```python
from build123d import *

# Parameters (mm, degrees)
SKETCH1_W                = 222.53
SKETCH1_H                = 140
TOP_PLATE_DEPTH          = 6
CORNER_FILLET_R          = 5
M3_CLEARANCE_HOLE1_D     = 3.4
M3_CLEARANCE_HOLE1_DEPTH = 4.228536948
M3_CLEARANCE_HOLE1_TIP   = 1.021463052
SKETCH4_R                = 16.25
SKETCH4_R_2              = 13.25
PRIMARY_BUTTONS_DEPTH    = 10
EXTRA_BUTTONS_REACH      = 8
SKETCH8_W                = 207.53
SKETCH8_H                = 125
HOLLOW_OUT_DEPTH         = 3.3
FILLET1_R                = 10
FILLET2_R                = 5
SKETCH15_W               = 64
SKETCH15_H               = 16
CUT_EXTRUDE4_DEPTH       = 4.4
LIGHT_GUIDE_CUTOUT_DEPTH = 10
CHAMFER1_SIZE            = 1
TOP_CHAMFER_SIZE         = 1.5
NUT_START                = -1.2
NUT_CUTOUT_DEPTH         = 2


with BuildPart() as part:
    # Sketch1 → Top Plate (new body)
    with BuildSketch(Plane(origin=(0, 0, 0), x_dir=(1, 0, 0), z_dir=(0, 1, 0))):
        with Locations((111.265, 70)):
            Rectangle(SKETCH1_W, SKETCH1_H)
    extrude(amount=TOP_PLATE_DEPTH)

    # Corner Fillet
    corner_fillet_edges = [part.edges().sort_by_distance(p)[0] for p in [
        (0, 3, -140),
        (222.53, 3, -140),
        (222.53, 3, 0),
        (0, 3, 0),
    ]]
    fillet(corner_fillet_edges, radius=CORNER_FILLET_R)

    # M3 Clearance Hole1
    with Locations(Plane(origin=(217.03, 0, -5.5), x_dir=(0, 0, -1), z_dir=(0, -1, 0))):
        with Locations((0, 0), (129, 0), (129, -211.53), (0, -211.53)):
            Hole(M3_CLEARANCE_HOLE1_D / 2, depth=M3_CLEARANCE_HOLE1_DEPTH)
            with Locations((0, 0, -(M3_CLEARANCE_HOLE1_DEPTH + M3_CLEARANCE_HOLE1_TIP / 2))):  # 118° drill point
                Cone(0, M3_CLEARANCE_HOLE1_D / 2, M3_CLEARANCE_HOLE1_TIP, mode=Mode.SUBTRACT)

    # Sketch4 → Primary Buttons (cut)
    with BuildSketch(Plane(origin=(0, 6, 0), x_dir=(-1, 0, 0), z_dir=(0, -1, 0))):
        with BuildLine():
            ThreePointArc((-48.971318984, 103.179989332), (-49.620754304, 103.829424652), (-50.539194542, 103.829424652))
            Line((-50.539194542, 103.829424652), (-67.030443813, 96.998525544))
            Line((-67.030443813, 96.998525544), (-73.861342517, 113.489775595))
            ThreePointArc((-73.861342517, 113.489775595), (-74.510777833, 114.139210949), (-75.429218092, 114.139210957))
            Line((-75.429218092, 114.139210957), (-93.029123186, 106.849091571))
            ThreePointArc((-93.029123186, 106.849091571), (-93.678558502, 106.199656261), (-93.678558515, 105.281216033))
            Line((-93.678558515, 105.281216033), (-86.388439374, 87.681310625))
            Line((-86.388439374, 87.681310625), (-85.316925644, 85.094447645))
            Line((-85.316925644, 85.094447645), (-101.80817536, 78.263548352))
            ThreePointArc((-101.80817536, 78.263548352), (-102.457610681, 77.614113031), (-102.457610681, 76.695672794))
            Line((-102.457610681, 76.695672794), (-95.167491294, 59.095767699))
            ThreePointArc((-95.167491294, 59.095767699), (-94.518055974, 58.446332379), (-93.599615736, 58.446332379))
            Line((-93.599615736, 58.446332379), (-75.999710782, 65.736451708))
            ThreePointArc((-75.999710782, 65.736451708), (-75.350275462, 66.385887028), (-75.350275462, 67.304327265))
            Line((-75.350275462, 67.304327265), (-76.421789326, 69.891190568))
            Line((-76.421789326, 69.891190568), (-59.93053937, 76.722089559))
            Line((-59.93053937, 76.722089559), (-42.330634918, 84.01220868))
            ThreePointArc((-42.330634918, 84.01220868), (-41.681199598, 84.661644), (-41.681199598, 85.580084238))
            Line((-41.681199598, 85.580084238), (-48.971318984, 103.179989332))
        make_face()
        with Locations((-23, 83.008304)):
            Circle(SKETCH4_R)
        with Locations((-112.915906, 94.645876)):
            Circle(SKETCH4_R_2)
        with Locations((-138.114257, 108.999439)):
            Circle(SKETCH4_R_2)
        with Locations((-162.933943, 94)):
            Circle(SKETCH4_R_2)
        with Locations((-191.933943, 94)):
            Circle(SKETCH4_R_2)
        with Locations((-137.933943, 80)):
            Circle(SKETCH4_R_2)
        with Locations((-137.933943, 51)):
            Circle(SKETCH4_R_2)
        with Locations((-162.933943, 65)):
            Circle(SKETCH4_R_2)
        with Locations((-191.933943, 65)):
            Circle(SKETCH4_R_2)
        with BuildLine():
            ThreePointArc((-102.903943224, 5.899999517), (-89.803943224, 18.999999517), (-102.903943224, 32.099999517))
            Line((-102.903943224, 32.099999517), (-123.903943224, 32.099999517))
            ThreePointArc((-123.903943224, 32.099999517), (-137.003943224, 18.999999517), (-123.903943224, 5.899999517))
            Line((-123.903943224, 5.899999517), (-102.903943224, 5.899999517))
        make_face()
    extrude(amount=PRIMARY_BUTTONS_DEPTH, mode=Mode.SUBTRACT)

    # Sketch5 → Extra Buttons (cut, up to next)
    with BuildSketch(Plane.XZ, mode=Mode.PRIVATE) as extra_buttons_sk1:
        with BuildLine():
            Line((154.55, -122.52), (154.55, -117.32))
            ThreePointArc((154.55, -117.32), (154.842893219, -116.612893219), (155.55, -116.32))
            Line((155.55, -116.32), (163.05, -116.32))
            ThreePointArc((163.05, -116.32), (163.757106781, -116.612893219), (164.05, -117.32))
            Line((164.05, -117.32), (164.05, -122.52))
            ThreePointArc((164.05, -122.52), (163.757106781, -123.227106781), (163.05, -123.52))
            Line((163.05, -123.52), (155.55, -123.52))
            ThreePointArc((155.55, -123.52), (154.842893219, -123.227106781), (154.55, -122.52))
        make_face()
    extra_buttons_tool1 = extrude(extra_buttons_sk1.sketch, amount=-EXTRA_BUTTONS_REACH, mode=Mode.PRIVATE) & part.part
    add(extra_buttons_tool1.solids().sort_by_distance((159.3, 0, -119.92))[0], mode=Mode.SUBTRACT)
    # Sketch5 → Extra Buttons (cut, up to next)
    with BuildSketch(Plane.XZ, mode=Mode.PRIVATE) as extra_buttons_sk2:
        with BuildLine():
            Line((170.55, -122.52), (170.55, -117.32))
            ThreePointArc((170.55, -117.32), (170.842893219, -116.612893219), (171.55, -116.32))
            Line((171.55, -116.32), (179.05, -116.32))
            ThreePointArc((179.05, -116.32), (179.757106781, -116.612893219), (180.05, -117.32))
            Line((180.05, -117.32), (180.05, -122.52))
            ThreePointArc((180.05, -122.52), (179.757106781, -123.227106781), (179.05, -123.52))
            Line((179.05, -123.52), (171.55, -123.52))
            ThreePointArc((171.55, -123.52), (170.842893219, -123.227106781), (170.55, -122.52))
        make_face()
    extra_buttons_tool2 = extrude(extra_buttons_sk2.sketch, amount=-EXTRA_BUTTONS_REACH, mode=Mode.PRIVATE) & part.part
    add(extra_buttons_tool2.solids().sort_by_distance((175.3, 0, -119.92))[0], mode=Mode.SUBTRACT)
    # Sketch5 → Extra Buttons (cut, up to next)
    with BuildSketch(Plane.XZ, mode=Mode.PRIVATE) as extra_buttons_sk3:
        with BuildLine():
            Line((186.55, -122.52), (186.55, -117.32))
            ThreePointArc((186.55, -117.32), (186.842893219, -116.612893219), (187.55, -116.32))
            Line((187.55, -116.32), (195.05, -116.32))
            ThreePointArc((195.05, -116.32), (195.757106781, -116.612893219), (196.05, -117.32))
            Line((196.05, -117.32), (196.05, -122.52))
            ThreePointArc((196.05, -122.52), (195.757106781, -123.227106781), (195.05, -123.52))
            Line((195.05, -123.52), (187.55, -123.52))
            ThreePointArc((187.55, -123.52), (186.842893219, -123.227106781), (186.55, -122.52))
        make_face()
    extra_buttons_tool3 = extrude(extra_buttons_sk3.sketch, amount=-EXTRA_BUTTONS_REACH, mode=Mode.PRIVATE) & part.part
    add(extra_buttons_tool3.solids().sort_by_distance((191.3, 0, -119.92))[0], mode=Mode.SUBTRACT)
    # Sketch5 → Extra Buttons (cut, up to next)
    with BuildSketch(Plane.XZ, mode=Mode.PRIVATE) as extra_buttons_sk4:
        with BuildLine():
            Line((202.55, -122.52), (202.55, -117.32))
            ThreePointArc((202.55, -117.32), (202.842893219, -116.612893219), (203.55, -116.32))
            Line((203.55, -116.32), (211.05, -116.32))
            ThreePointArc((211.05, -116.32), (211.757106781, -116.612893219), (212.05, -117.32))
            Line((212.05, -117.32), (212.05, -122.52))
            ThreePointArc((212.05, -122.52), (211.757106781, -123.227106781), (211.05, -123.52))
            Line((211.05, -123.52), (203.55, -123.52))
            ThreePointArc((203.55, -123.52), (202.842893219, -123.227106781), (202.55, -122.52))
        make_face()
    extra_buttons_tool4 = extrude(extra_buttons_sk4.sketch, amount=-EXTRA_BUTTONS_REACH, mode=Mode.PRIVATE) & part.part
    add(extra_buttons_tool4.solids().sort_by_distance((207.3, 0, -119.92))[0], mode=Mode.SUBTRACT)

    # Sketch8 → Hollow Out (cut)
    with BuildSketch(Plane.XZ):
        with Locations((111.265, -70)):
            Rectangle(SKETCH8_W, SKETCH8_H)
    extrude(amount=-HOLLOW_OUT_DEPTH, mode=Mode.SUBTRACT)

    # Fillet1
    fillet1_edges = [part.edges().sort_by_distance(p)[0] for p in [
        (7.5, 1.65, -7.5),
        (7.5, 1.65, -132.5),
        (215.03, 1.65, -7.5),
    ]]
    fillet(fillet1_edges, radius=FILLET1_R)

    # Fillet2
    fillet2_edges = [part.edges().sort_by_distance(p)[0] for p in [
        (215.03, 1.65, -132.5),
    ]]
    fillet(fillet2_edges, radius=FILLET2_R)

    # Sketch15 → Cut-Extrude4 (cut)
    with BuildSketch(Plane.XZ):
        with Locations((183.3, -119.92)):
            Rectangle(SKETCH15_W, SKETCH15_H)
    extrude(amount=-CUT_EXTRUDE4_DEPTH, mode=Mode.SUBTRACT)

    # Sketch9 → Light Guide Cutout (cut)
    with BuildSketch(Plane(origin=(0, 6, 0), x_dir=(1, 0, 0), z_dir=(0, 1, 0))):
        with BuildLine():
            Line((65.42, 125.5875), (73.19, 125.5875))
            ThreePointArc((73.19, 125.5875), (77.19, 121.5875), (73.19, 117.5875))
            Line((73.19, 117.5875), (65.42, 117.5875))
            ThreePointArc((65.42, 117.5875), (61.42, 121.5875), (65.42, 125.5875))
        make_face()
    extrude(amount=-LIGHT_GUIDE_CUTOUT_DEPTH, mode=Mode.SUBTRACT)

    # Chamfer1
    chamfer1_edges = [part.edges().sort_by_distance(p)[0] for p in [
        (69.305, 3.3, -117.5875),
        (77.19, 3.3, -121.5875),
        (69.305, 3.3, -125.5875),
        (61.42, 3.3, -121.5875),
    ]]
    chamfer(chamfer1_edges, length=CHAMFER1_SIZE)

    # Top Chamfer
    top_chamfer_edges = [part.edges().sort_by_distance(p)[0] for p in [
        (0, 6, -70),
        (111.265, 6, -140),
        (111.265, 6, 0),
        (222.53, 6, -70),
        (221.065533906, 6, -1.464466094),
        (221.065533906, 6, -138.535533906),
        (1.464466094, 6, -1.464466094),
        (1.464466094, 6, -138.535533906),
    ]]
    chamfer(top_chamfer_edges, length=TOP_CHAMFER_SIZE)

    # Sketch11 → Nut Cutout (cut)
    with BuildSketch(Plane.XZ.offset(NUT_START)):
        Polygon((217.03, -138.601219331), (212.928780669, -134.5), (217.03, -130.398780669), (221.131219331, -134.5), align=None)
        Polygon((1.398780669, -134.5), (5.5, -130.398780669), (9.601219331, -134.5), (5.5, -138.601219331), align=None)
        Polygon((5.5, -9.601219331), (1.398780669, -5.5), (5.5, -1.398780669), (9.601219331, -5.5), align=None)
        Polygon((217.03, -9.601219331), (212.928780669, -5.5), (217.03, -1.398780669), (221.131219331, -5.5), align=None)
    extrude(amount=-NUT_CUTOUT_DEPTH, mode=Mode.SUBTRACT)


solid = part.part
```
For this review, take the finished solid that the model builds, in its own axes (mm). A direction names the side the tool comes from. Round coordinates to 2 decimals unless told otherwise and drop trailing zeros. Loops run counter-clockwise (first coordinate to the right, second up) from the corner with the lowest first, then second, coordinate; pieces in that order, holes last.
(1) Clearance check with flat-ended pins moving along their axes: P1, Ø0.5, axis at x = 206, y = 5.5, coming from the -Z side; P2, Ø0.8, axis at x = 71, y = 5.5, coming from the +Z side; P3, Ø0.8, axis at x = 206, y = 5, coming from the +Z side. State where each tip first meets the part, or that it passes through.
Returned:
P1: stops at z = -139.25
P2: stops at z = -0.6
P3: stops at z = -0.1
(2) Mouldability with a two-part tool opening along Y and no side actions: class faces 1 (the flat face through (58.67, 4.67, -100.46)), 2 (the flat face through (215.01, 2.19, -136.58)) as released by +Y, released by -Y, zero draft, split by the parting line, or undercut.
Returned:
face 1: zero draft
face 2: undercut
(3) Wall thickness on line 1 along Z through (x, y) = (217.03, 0.55); line 2 along X through (y, z) = (1, -114); line 3 along Z through (x, y) = (103.5, 1.5): over which ranges is each line inside the solid? List them lowest first.
Returned:
line 1: z = -140 to -136.2, -132.8 to -7.2, -3.8 to 0
line 2: x = 0 to 7.5, 215.3 to 222.53
line 3: z = -140 to -132.5, -5.9 to 0
(4) Tool access review of faces 3 (the flat face through (110, 2, -140)), 4 (the flat face through (214.95, 2.19, -132.48)), 5 (the cylindrical face through (213.5, 1.7, -131.1)), 6 (the flat face through (114, 3, -5.9)): name each direction out of +Z, -Z, +X, -X, +Y, -Y from which nothing blocks a thin tool from reaching the whole face with its end or side.
Returned:
face 3: -Z, +X, -X, +Y, -Y
face 4: none
face 5: -Y
face 6: +Y, -Y
(5) We need section B-B (z = -29.5). Give the boundary of the cut face in (x, y), plus the area to 3 significant figures.
Returned:
outline: (0, 0) - (7.5, 0) - (7.5, 3.3) - (95.07, 3.3) - (95.07, 6) - (1.5, 6) - (0, 4.5) - close; (131.74, 3.3) - (215.03, 3.3) - (215.03, 0) - (222.53, 0) - (222.53, 4.5) - (221.03, 6) - (131.74, 6) - close
area: 549 mm2
(6) We need section A-A (x = 80.5). Give the boundary of the cut face in (y, z), plus the area to 3 significant figures.
Returned:
outline: (0, -140) - (4.5, -140) - (6, -138.5) - (6, -112.04) - (3.3, -112.04) - (3.3, -132.5) - (0, -132.5) - close; (0, -7.5) - (3.3, -7.5) - (3.3, -63.87) - (6, -63.87) - (6, -1.5) - (4.5, 0) - (0, 0) - close
area: 295 mm2
